Check sheet for the modelled part. Datum: model origin and axes. Units: mm. Coordinates: 2 decimals unless noted, no trailing zeros. Write each loop counter-clockwise with the first axis right and the second up, starting at its lowest first coordinate (ties: lowest second). Pieces come first, ordered by that corner, then holes. Notation, with made-up numbers: (-10, 69) -> (2, 69) arc R25 ccw to (2, 82) -> close; hole circle Ø6 at (-1.75, 41.25). An arc over 180 degrees is marked (long way). Put each result on its own line as item: value.
```python
from build123d import *

# Parameters (mm, degrees)
SKETCH1_W           = 12.7
SKETCH1_H           = 3.175
BOSS_EXTRUDE1_DEPTH = 3.175


with BuildPart() as part:
    # Sketch1 → Boss-Extrude1 (new body)
    with BuildSketch(Plane.XY):
        Polygon((152.4, 0), (152.4, 128.913945011), (133.35, 128.913945011), (133.35, 132.088945011), (101.6, 132.088945011), (101.6, 128.913945011), (82.55, 128.913945011), (82.55, 132.088945011), (45.481871178, 132.088945011), (37.212440054, 108.072773191), (40.214461532, 107.039094301), (34.01238819, 89.026965435), (31.010366712, 90.060644326), (24.80829337, 72.048515461), (27.810314847, 71.01483657), (21.608241505, 53.002707705), (18.606220027, 54.036386596), (12.404146685, 36.02425773), (15.406168162, 34.99057884), (9.20409482, 16.978449975), (6.202073342, 18.012128865), (0, 0), (9.97035014, -12.312357038), (12.437788568, -10.314264796), (24.426342017, -25.118895362), (21.95890359, -27.116987604), (41.939826006, -51.79137188), (44.407264433, -49.793279638), (56.395817883, -64.597910204), (53.928379455, -66.596002446), (55.946582764, -69.088275974), align=None)
        with Locations((88.9, 1.5875)):
            Rectangle(SKETCH1_W, SKETCH1_H, mode=Mode.SUBTRACT)
        with Locations((127, 1.5875)):
            Rectangle(SKETCH1_W, SKETCH1_H, mode=Mode.SUBTRACT)
        with Locations((50.8, 1.5875)):
            Rectangle(SKETCH1_W, SKETCH1_H, mode=Mode.SUBTRACT)
    extrude(amount=BOSS_EXTRUDE1_DEPTH)


solid = part.part
```
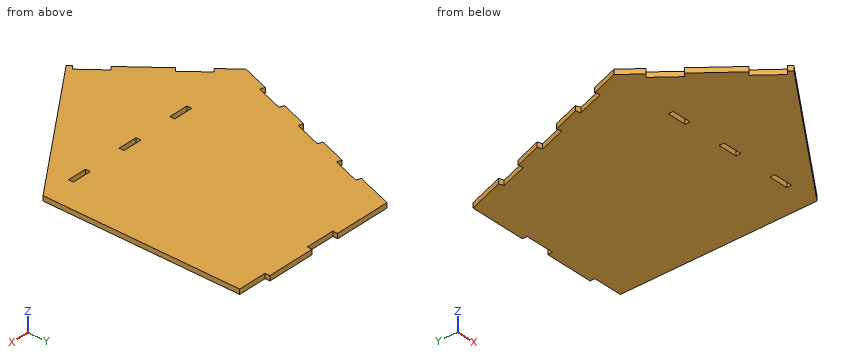
Q1. Cross-section at C-C (y = 42). Record the cut outline in (x, z) (3 decimals).
Recorded:
outline: (14.462, 0) -> (152.4, 0) -> (152.4, 3.175) -> (14.462, 3.175) -> close
Q2. Cross-section at D-D (x = 106.5). Record the cut outline in (y, z) (3 decimals), plus the area to 3 significant figures.
Recorded:
outline: (-32.878, 0) -> (132.089, 0) -> (132.089, 3.175) -> (-32.878, 3.175) -> close
area: 524 mm2
Q3. Cross-section at A-A (x = 48). Record the cut outline in (y, z) (3 decimals).
Recorded:
outline: (-54.23, 0) -> (0, 0) -> (0, 3.175) -> (-54.23, 3.175) -> close; (3.175, 0) -> (132.089, 0) -> (132.089, 3.175) -> (3.175, 3.175) -> close
Q4. Depth check by flat-ended pin: P1, Ø1, axis at y = 130.5, z = 1, coming from the +X side; P2, Ø1, axis at x = 87.5, z = 1.5, coming from the +Y side; P3, Ø1.6, axis at x = 88, z = 1, coming from the -Y side. Enter the tip coordinate at first touch or a pass-through.
Recorded:
P1: stops at x = 133.35
P2: stops at y = 128.91
P3: stops at y = -46.7
Q5. Material ranges on line 1 along Y through (x, z) = (89.5, 1.6) (3 decimals); line 2 along X through (y, z) = (87, 0.85); line 3 along Y through (x, z) = (86, 1.55) (3 decimals), recorded low to high.
Recorded:
line 1: y = -45.054 to 0, 3.175 to 128.914
line 2: x = 29.96 to 152.4
line 3: y = -47.561 to 0, 3.175 to 128.914
Q6. Cross-section at B-B (z = 1.95). State how many separate pieces and enclosed holes the cut face has, plus the area to 3 significant figures.
Recorded:
separate pieces: 1
enclosed holes: 3
area: 21,800 mm2
